from build123d import *

# Parameters (mm, degrees)
SKETCH2_W           = 15
SKETCH2_H           = 20
BOSS_EXTRUDE1_DEPTH = 8
SKETCH3_W           = 15
SKETCH3_H           = 5
BOSS_EXTRUDE4_DEPTH = 28
SKETCH6_W           = 15
SKETCH6_H           = 10
BOSS_EXTRUDE5_DEPTH = 6
SKETCH8_R           = 1.7
CUT_EXTRUDE1_DEPTH  = 44.084219849
CIRPATTERN1_COUNT   = 4
FILLET1_R           = 6
SKETCH9_R           = 1.7
CUT_EXTRUDE2_DEPTH  = 56.641710973


with BuildPart() as part:
    # Sketch2 → Boss-Extrude1 (new body)
    with BuildSketch(Plane(origin=(0, 0, 0), x_dir=(1, 0, 0), z_dir=(0, 1, 0))):
        with Locations((0, 10)):
            Rectangle(SKETCH2_W, SKETCH2_H)
    boss_extrude1 = extrude(amount=-BOSS_EXTRUDE1_DEPTH)

    # Sketch3 → Boss-Extrude4 (add)
    with BuildSketch(Plane(origin=(0, 0, 0), x_dir=(1, 0, 0), z_dir=(0, 1, 0))):
        with Locations((0, 17.5)):
            Rectangle(SKETCH3_W, SKETCH3_H)
    boss_extrude4 = extrude(amount=BOSS_EXTRUDE4_DEPTH)

    # Sketch6 → Boss-Extrude5 (add)
    with BuildSketch(Plane(origin=(0, 28, 0), x_dir=(1, 0, 0), z_dir=(0, 1, 0))):
        with Locations((0, 25)):
            Rectangle(SKETCH6_W, SKETCH6_H)
    boss_extrude5 = extrude(amount=-BOSS_EXTRUDE5_DEPTH)

    # Sketch8 → Cut-Extrude1 (cut, through all)
    with BuildSketch(Plane.XZ.offset(-22)):
        with Locations(Location((0, -25, 0), (0, 0, 270))):
            Circle(SKETCH8_R)
    cut_extrude1 = extrude(amount=-CUT_EXTRUDE1_DEPTH, mode=Mode.SUBTRACT)

    # CirPattern1: Boss-Extrude1, Boss-Extrude4, Boss-Extrude5, Cut-Extrude1 ×4 about axis
    cirpattern1_axis = Axis((0, 0, 0), (0, 1, 0))
    add([boss_extrude1.rotate(cirpattern1_axis, i * 360 / CIRPATTERN1_COUNT) for i in range(1, CIRPATTERN1_COUNT)])
    add([boss_extrude4.rotate(cirpattern1_axis, i * 360 / CIRPATTERN1_COUNT) for i in range(1, CIRPATTERN1_COUNT)])
    add([boss_extrude5.rotate(cirpattern1_axis, i * 360 / CIRPATTERN1_COUNT) for i in range(1, CIRPATTERN1_COUNT)])
    add([cut_extrude1.rotate(cirpattern1_axis, i * 360 / CIRPATTERN1_COUNT) for i in range(1, CIRPATTERN1_COUNT)], mode=Mode.SUBTRACT)

    # Fillet1
    fillet1_edges = [part.edges().sort_by_distance(p)[0] for p in [
        (-7.5, -4, -7.5),
        (7.5, -4, -7.5),
        (-7.5, -4, 7.5),
        (7.5, -4, 7.5),
    ]]
    fillet(fillet1_edges, radius=FILLET1_R)

    # Sketch9 → Cut-Extrude2 (cut, through all)
    with BuildSketch(Plane.XZ.offset(8)):
        with Locations(Location((0, 8, 0), (0, 0, 270))):
            Circle(SKETCH9_R)
        with Locations(Location((9.5, 0, 0), (0, 0, 270))):
            Circle(SKETCH9_R)
        with Locations(Location((0, -8, 0), (0, 0, 270))):
            Circle(SKETCH9_R)
        with Locations(Location((-9.5, 0, 0), (0, 0, 270))):
            Circle(SKETCH9_R)
    extrude(amount=-CUT_EXTRUDE2_DEPTH, mode=Mode.SUBTRACT)


solid = part.part
Geometry: final body of the model. Coordinates: model frame, mm. A direction names the side the tool comes from. Coordinates: 2 decimals unless noted, no trailing zeros. Order: outer loops, then holes, each group sorted by start corner. A loop starts at its lowest first (then second) coordinate and runs counter-clockwise, first axis right, second up. Notation, with made-up numbers: M 17,27.25 L 49,27.25 A20 ccw 49,53.25 Z; hole C -30.75,13.5 d9. An arc over 180 degrees is marked long. One line per question, with ' | ' between items. Start each with the question number.
Item 1: Set-up query: faces 1 (the flat face through (-19.8, 14.3, 7.5)), 2 (the flat face through (-7.5, 14.3, -19.8)), 3 (the flat face through (-25, 22, 2)), 4 (the flat face through (0, 14, 15)), 5 (the flat face through (19.8, 14.3, 7.5)). Return all of +Z, -Z, +X, -X, +Y, -Y with unobstructed straight access to the full face (end or side cutting, diameter ignored); none if empty.
Item 2: Cut plane A-A, the plane x = 0. Return the cut outline in (y, z).
Item 3: Cut plane D-D, the plane x = 25. Return the cut outline in (y, z).
Item 4: Cut plane C-C, the plane y = -2.5. Return the cut outline in (x, z), then the cut area to 3 significant figures.
Item 5: Ray query, probe 1 along X at (y, z) = (-4, 0); probe 2 along Z at (x, y) = (3, 2.5); probe 3 along Z at (x, y) = (4, 24). Return the intervals inside material, ascending. Write a range as [from, to].
Item 6: Pin query (flat end, axial travel): pin 1 Ø18 at (x, y) = (18.5, 11.5) entering from -Z; pin 2 Ø4 at (x, z) = (0, 8) entering from +Y; pin 3 Ø5 at (x, z) = (1.5, 25) entering from -Y; pin 4 Ø4 at (x, y) = (22.5, 9) entering from +Z. Return the tip coordinate at first contact, or that it passes through.
Item 7: Cut plane B-B, the plane z = 0. Return the cut outline in (x, y).
Item 8: Draft query along X for faces 6 (the flat face through (7.5, 14.3, -19.8)), 7 (the cylindrical face through (-11.16, -4.06, 0.37)), 8 (the flat face through (-20, 7, 0)), 9 (the flat face through (-19.8, 14.3, -7.5)). Return one class per face: released by +X, released by -X, zero draft, split by the parting line, or undercut.
A:
1) face 1: +Z, -X, +Y, -Y | face 2: -Z, -X, +Y, -Y | face 3: +Z, -Z, -X, -Y | face 4: +X, -X, +Y | face 5: +Z, +X, +Y, -Y
2) outline: M -8,-20 L 22,-20 L 22,-23.3 L 28,-23.3 L 28,-15 L 0,-15 L 0,-9.7 L -8,-9.7 Z; M -8,-6.3 L 0,-6.3 L 0,6.3 L -8,6.3 Z; M -8,9.7 L 0,9.7 L 0,15 L 28,15 L 28,23.3 L 22,23.3 L 22,20 L -8,20 Z; M 22,-30 L 28,-30 L 28,-26.7 L 22,-26.7 Z; M 22,26.7 L 28,26.7 L 28,30 L 22,30 Z
3) outline: M 22,-7.5 L 28,-7.5 L 28,-1.7 L 22,-1.7 Z; M 22,1.7 L 28,1.7 L 28,7.5 L 22,7.5 Z
4) outline: M -20,-7.5 L -13.5,-7.5 A6 cw -7.5,-13.5 L -7.5,-20 L 7.5,-20 L 7.5,-13.5 A6 cw 13.5,-7.5 L 20,-7.5 L 20,7.5 L 13.5,7.5 A6 cw 7.5,13.5 L 7.5,20 L -7.5,20 L -7.5,13.5 A6 cw -13.5,7.5 L -20,7.5 Z; hole C -9.5,0 d3.4; hole C 0,-8 d3.4; hole C 0,8 d3.4; hole C 9.5,0 d3.4 | area: 970 mm2
5) probe 1: x = [-20, -11.2], [-7.8, 7.8], [11.2, 20] | probe 2: z = [-20, -15], [15, 20] | probe 3: z = [-30, -15], [15, 30]
6) pin 1: stops at z = -7.5 | pin 2: stops at y = 0 | pin 3: stops at y = 22 | pin 4: passes through
7) outline: M -30,22 L -26.7,22 L -26.7,28 L -30,28 Z; M -23.3,22 L -20,22 L -20,-8 L -11.2,-8 L -11.2,0 L -15,0 L -15,28 L -23.3,28 Z; M -7.8,-8 L 7.8,-8 L 7.8,0 L -7.8,0 Z; M 11.2,-8 L 20,-8 L 20,22 L 23.3,22 L 23.3,28 L 15,28 L 15,0 L 11.2,0 Z; M 26.7,22 L 30,22 L 30,28 L 26.7,28 Z
8) face 6: released by +X | face 7: undercut | face 8: released by -X | face 9: zero draft
